The listing builds one solid part. Answer for the finished solid, in the listing's coordinates (mm). A direction names the side the tool comes from. Give positions to 0.01 mm unless a question says otherwise; leave off trailing zeros. Write each loop counter-clockwise with the first axis right and the second up, starting at its lowest first coordinate (ties: lowest second). Pieces come first, ordered by that corner, then holes. Notation, with made-up numbers: M 76.25,84.25 L 118.25,84.25 A12 ccw 118.25,93.25 Z; hole C 8,49.5 d10. An arc over 180 degrees is marked long. Answer as a JSON object with one key per item and string values.
Autodesk Inventor part; units mm, degrees
ref_plane "YZ Plane" through (0, 0, 0) normal (1, 0, 0) x (0, 1, 0)
ref_plane "XZ Plane" through (0, 0, 0) normal (0, 1, 0) x (-1, 0, 0)
ref_plane "XY Plane" through (0, 0, 0) normal (0, 0, 1) x (1, 0, 0)
sketch "Sketch1" plane through (0, 0, 0) normal (0, 0, 1) x (1, 0, 0)
  line L0 (-39.1795, 4.7625) -> (39.1795, 4.7625)
  line L1 (39.1795, 4.7625) -> (39.1795, -4.7625)
  line L2 (39.1795, -4.7625) -> (-39.1795, -4.7625)
  line L3 (-39.1795, -4.7625) -> (-39.1795, 4.7625)
  line L4 (-39.1795, 4.7625) -> (39.1795, -4.7625) construction
  line L5 (39.1795, 4.7625) -> (-39.1795, -4.7625) construction
  point P0 (0, 0)
  dimension "d0" = 78.359
  dimension "d1" = 9.525
extrude "Extrusion1" add sketch "Sketch1" along normal blind 3.175
sketch "Sketch2" plane through (0, 0, 0) normal (0, 0, -1) x (-1, 0, 0)
  line L0 (-54.8513, 0) -> (54.8513, 0)
  line L1 (0, -6.6675) -> (0, 6.6675)
  line L2 (39.1795, -4.7625) -> (-39.1795, -4.7625)
  line L3 (39.1795, 4.7625) -> (39.1795, -4.7625)
  line L4 (-39.1795, 4.7625) -> (39.1795, 4.7625)
  line L5 (-39.1795, -4.7625) -> (-39.1795, 4.7625)
  circle A0 centre (0, 2.6797) radius 1.5875
  point P0 (0, 0)
  dimension "d4" = 3.175
  dimension "d5" = 2.0828
extrude "Extrusion2" cut sketch "Sketch2" against normal blind 0.7937 contours A0 L1 | L1 A0
pattern_linear "Rectangular Pattern1" count 11 spacing 6.35 along (1, 0, 0) of "Extrusion2" first direction both ways yes
equation "\"BendRadius\" = Thickness"
equation "\"BendReliefWidth\" = Thickness"
equation "\"BendReliefDepth\" = 0.5 * Thickness"
equation "\"CornerReliefSize\" = 4 * Thickness"
equation "\"MinimumRemnant\" = 2 * Thickness"
equation "\"TransitionRadius\" = BendRadius"
equation "\"JacobiRadiusSize\" = BendRadius"
equation "\"GapSize\" = Thickness"
properties part number "PrintHeadLoadPlate"
1. A flat-ended cylindrical pin translates along its axis: pin 1 (3 mm diameter, centred on x = -19.05, y = 2.68, fed in from -Z). Find the tip coordinate at first contact, or state that the pin passes through.
Verdict:
{"pin 1": "stops at z = 0.79"}
2. For faces 3 (the flat face through (-1, 0, 3.175)), 4 (the flat face through (25, 3, 0.794)), determine the directions among +Z, -Z, +X, -X, +Y, -Y from which every point of the face is accessible in a straight line to the end or side of a thin tool.
Verdict:
{"face 3": "+Z, +X, -X, +Y, -Y", "face 4": "-Z"}
3. The mould has two halves that part along X. Classify faces 1 (the flat face through (19, 3, 0.794)), 2 (the flat face through (-1, 0, 0)): released by +X, released by -X, zero draft, split by the parting line, or undercut.
Verdict:
{"face 1": "undercut", "face 2": "zero draft"}
4. Consider line 1 along Y through (x, z) = (-12.7, 0.5); line 2 along Z through (x, y) = (-6, 3.5) (3 decimals). Determine where each line is inside the solid, lowest interval first.
Verdict:
{"line 1": "y = -4.76 to 1.09, 4.27 to 4.76", "line 2": "z = 0.794 to 3.175"}
5. A cutting plane is placed at A-A, the plane x = -19.05. Give the vertices of the cut face in (y, z) (1 decimal).
Verdict:
{"outline": "M -4.8,0 L 1.1,0 L 1.1,0.8 L 4.3,0.8 L 4.3,0 L 4.8,0 L 4.8,3.2 L -4.8,3.2 Z"}
